Check sheet for the modelled part. Datum: model origin and axes. Units: mm. Round coordinates to 2 decimals unless told otherwise and drop trailing zeros. Loops run counter-clockwise (first coordinate to the right, second up) from the corner with the lowest first, then second, coordinate; pieces in that order, holes last. Notation, with made-up numbers: (-26.5, -39) - (-13.5, -39) arc R16 cw to (-13.5, -31) - close; hole circle Ø7 at (83, -17.75). An arc over 180 degrees is marked (long way). Answer in a Markdown table with one row per item. Add a question column.
(1) Gauge pin test, flat ends, axial feed: pin 1 (2.5 mm diameter, centred on x = -17.84, z = -1.27, fed in from -Y); pin 2 (1 mm diameter, centred on y = 2.5, z = 19.5, fed in from -X). Record the tip position at first contact, or that the pin passes through.
(2) Cross-section at C-C on y = 2.25. Count the separate pieces of the cut face and the enclosed holes in it, then the cut area to 3 significant figures.
(3) Cross-section at B-B on z = 20. Enter the section's corners in (x, y).
(4) Thickness scan on line 1 along Z through (x, y) = (-26.5, 1.2); line 2 along X through (y, z) = (0.55, 19); line 3 along Z through (x, y) = (1.5, 2.65). Record the ranges inside material, lowest first.
(5) Mould release check, pull along X, two halves, no side actions. Record for faces 1 (the cylindrical face through (0.049, 1.479, 11.293)), 2 (the flat face through (19.009, 1.479, -5.115)), 3 (the flat face through (-18.526, 1.479, -5.315)), 4 (the flat face through (-1, 3, 6)): +X half, -X half, draft (parallel to the pull), parting line (faces both ways), or undercut.
(6) Cross-section at A-A on z = 6. Enter the section's corners in (x, y).
from build123d import *

# Parameters (mm, degrees)
SKETCH1_R           = 2
SKETCH1_R_2         = 4
BOSS_EXTRUDE1_DEPTH = 3


with BuildPart() as part:
    # Sketch1 → Boss-Extrude1 (new body)
    with BuildSketch(Plane(origin=(0, 0, 0), x_dir=(1, 0, 0), z_dir=(0, 1, 0))):
        with BuildLine():
            ThreePointArc((1.530733729, 12.354655732), (0, 12.659137602), (-1.530733729, 12.354655732))
            Line((-1.530733729, 12.354655732), (-36.004105294, -1.92468231))
            ThreePointArc((-36.004105294, -1.92468231), (-37.086497494, -3.007074511), (-37.086497494, -4.53780824))
            Line((-37.086497494, -4.53780824), (-29.432828847, -23.01539889))
            ThreePointArc((-29.432828847, -23.01539889), (-28.350436646, -24.097791091), (-26.819702917, -24.097791091))
            Line((-26.819702917, -24.097791091), (-0.765366865, -13.305731739))
            ThreePointArc((-0.765366865, -13.305731739), (0, -13.153490804), (0.765366865, -13.305731739))
            Line((0.765366865, -13.305731739), (26.819702917, -24.097791091))
            ThreePointArc((26.819702917, -24.097791091), (28.350436646, -24.097791091), (29.432828847, -23.01539889))
            Line((29.432828847, -23.01539889), (37.086497494, -4.53780824))
            ThreePointArc((37.086497494, -4.53780824), (37.086497494, -3.007074511), (36.004105294, -1.92468231))
            Line((36.004105294, -1.92468231), (1.530733729, 12.354655732))
        make_face()
        with BuildLine():
            ThreePointArc((-9.452503719, 2.597517994), (-9.567926339, 2.535823318), (-9.687136854, 2.481809736))
            ThreePointArc((-9.687136854, 2.481809736), (-12.246249202, 3.444991421), (-11.452503719, 6.061619609))
            ThreePointArc((-11.452503719, 6.061619609), (0, 9.130308732), (11.452503719, 6.061619609))
            ThreePointArc((11.452503719, 6.061619609), (12.184554527, 3.329568801), (9.452503719, 2.597517994))
            ThreePointArc((9.452503719, 2.597517994), (4.892975973, 4.486136224), (0, 5.130308732))
            ThreePointArc((0, 5.130308732), (-4.892975973, 4.486136224), (-9.452503719, 2.597517994))
        make_face(mode=Mode.SUBTRACT)
        with Locations(Location((-26.502677581, -19.636906096, 0), (0, 0, 270))):
            Circle(SKETCH1_R, mode=Mode.SUBTRACT)
        with Locations(Location((-19.111641321, -16.575438637, 0), (0, 0, 270))):
            Circle(SKETCH1_R, mode=Mode.SUBTRACT)
        with Locations(Location((-29.56414504, -12.245869836, 0), (0, 0, 270))):
            Circle(SKETCH1_R, mode=Mode.SUBTRACT)
        with Locations(Location((-22.17310878, -9.184402377, 0), (0, 0, 270))):
            Circle(SKETCH1_R_2, mode=Mode.SUBTRACT)
        with Locations(Location((-11.720605061, -13.513971178, 0), (0, 0, 270))):
            Circle(SKETCH1_R, mode=Mode.SUBTRACT)
        with Locations(Location((-14.78207252, -6.122934918, 0), (0, 0, 270))):
            Circle(SKETCH1_R, mode=Mode.SUBTRACT)
        with BuildLine():
            ThreePointArc((-3.329568801, -12.184554527), (-6.061619609, -11.452503719), (-5.329568801, -8.720452911))
            ThreePointArc((-5.329568801, -8.720452911), (0, -7.292399255), (5.329568801, -8.720452911))
            ThreePointArc((5.329568801, -8.720452911), (6.061619609, -11.452503719), (3.329568801, -12.184554527))
            ThreePointArc((3.329568801, -12.184554527), (0, -11.292399255), (-3.329568801, -12.184554527))
        make_face(mode=Mode.SUBTRACT)
        with Locations(Location((26.502677581, -19.636906096, 0), (0, 0, 270))):
            Circle(SKETCH1_R, mode=Mode.SUBTRACT)
        with Locations(Location((19.111641321, -16.575438637, 0), (0, 0, 270))):
            Circle(SKETCH1_R, mode=Mode.SUBTRACT)
        with Locations(Location((11.720605061, -13.513971178, 0), (0, 0, 270))):
            Circle(SKETCH1_R, mode=Mode.SUBTRACT)
        with Locations(Location((14.78207252, -6.122934918, 0), (0, 0, 270))):
            Circle(SKETCH1_R, mode=Mode.SUBTRACT)
        with Locations(Location((29.56414504, -12.245869836, 0), (0, 0, 270))):
            Circle(SKETCH1_R, mode=Mode.SUBTRACT)
        with Locations(Location((22.17310878, -9.184402377, 0), (0, 0, 270))):
            Circle(SKETCH1_R_2, mode=Mode.SUBTRACT)
        with Locations(Location((-32.625612499, -4.854833576, 0), (0, 0, 270))):
            Circle(SKETCH1_R, mode=Mode.SUBTRACT)
        with Locations(Location((-25.234576239, -1.793366117, 0), (0, 0, 270))):
            Circle(SKETCH1_R, mode=Mode.SUBTRACT)
        with Locations(Location((-7.39103626, -3.061467459, 0), (0, 0, 270))):
            Circle(SKETCH1_R, mode=Mode.SUBTRACT)
        with Locations(Location((-17.843539979, 1.268101342, 0), (0, 0, 270))):
            Circle(SKETCH1_R, mode=Mode.SUBTRACT)
        with Locations(Location((0, 0, 0), (0, 0, 270))):
            Circle(SKETCH1_R, mode=Mode.SUBTRACT)
        with Locations(Location((7.39103626, -3.061467459, 0), (0, 0, 270))):
            Circle(SKETCH1_R, mode=Mode.SUBTRACT)
        with Locations(Location((25.234576239, -1.793366117, 0), (0, 0, 270))):
            Circle(SKETCH1_R, mode=Mode.SUBTRACT)
        with Locations(Location((32.625612499, -4.854833576, 0), (0, 0, 270))):
            Circle(SKETCH1_R, mode=Mode.SUBTRACT)
    extrude(amount=BOSS_EXTRUDE1_DEPTH)


solid = part.part
Answers:
| question | item | result |
|---|---|---|
| 1 | pin 1 | passes through |
| 1 | pin 2 | stops at x = -31.1 |
| 2 | separate pieces | 1 |
| 2 | enclosed holes | 22 |
| 2 | area | 1,250 mm^2 |
| 3 | outline | (-30.68, 0) - (-28.47, 0) - (-28.47, 3) - (-30.68, 3) - close; (-24.54, 0) - (-16.93, 0) - (-16.93, 3) - (-24.54, 3) - close; (16.93, 0) - (24.54, 0) - (24.54, 3) - (16.93, 3) - close; (28.47, 0) - (30.68, 0) - (30.68, 3) - (28.47, 3) - close |
| 4 | line 1 | z = -2.01 to 0.24, 3.34 to 17.64, 21.64 to 23.97 |
| 4 | line 2 | x = -31.1 to -28.4, -24.61 to -14.51, 14.51 to 24.61, 28.4 to 31.1 |
| 4 | line 3 | z = -12.37 to -9.08, -5.07 to -1.32, 1.32 to 7.4, 11.46 to 13.61 |
| 5 | face 1 | undercut |
| 5 | face 2 | +X half |
| 5 | face 3 | -X half |
| 5 | face 4 | draft |
| 6 | outline | (-36.48, 0) - (-34.27, 0) - (-34.27, 3) - (-36.48, 3) - close; (-30.99, 0) - (-24.59, 0) - (-24.59, 3) - (-30.99, 3) - close; (-19.75, 0) - (-16.78, 0) - (-16.78, 3) - (-19.75, 3) - close; (-12.79, 0) - (12.79, 0) - (12.79, 3) - (-12.79, 3) - close; (16.78, 0) - (19.75, 0) - (19.75, 3) - (16.78, 3) - close; (24.59, 0) - (30.99, 0) - (30.99, 3) - (24.59, 3) - close; (34.27, 0) - (36.48, 0) - (36.48, 3) - (34.27, 3) - close |
